Geometry check sheet. Reference: the model listing, model coordinates, mm. Face numbers are marked on the shaded views. A direction names the side the tool comes from. Give positions to 0.01 mm unless a question says otherwise; leave off trailing zeros. Loops run counter-clockwise (first coordinate to the right, second up) from the corner with the lowest first, then second, coordinate; pieces in that order, holes last. Notation, with made-up numbers: (62.25, -37.5) -> (82.25, -37.5) arc R20 cw to (82.25, -21.5) -> close; hole circle Ø10 at (60, 2). An arc over 180 degrees is marked (long way). One line per item, written item: value. Start each with the question number.
(1) Sectioned sample at C-C, the plane y = 42. Record the cut outline in (x, z).
(2) Sectioned sample at A-A, the plane x = 0. Record the cut outline in (y, z).
(3) Tool access check on the marked faces 1, 2 and 3. Record the directions out of +Z, -Z, +X, -X, +Y, -Y that give a thin tool (end or side, any length) a straight path to the whole face; none if there is none.
(4) Sectioned sample at B-B, the plane z = 0. Record the cut outline in (x, y).
(5) Scan lines: line 1 along Y through (x, z) = (6, -2.5); line 2 along X through (y, z) = (71.5, 0); line 3 along Y through (x, z) = (-3.5, -4). Record each from-to range of solid material in increasing order. Write a range as from..to.
(6) Sectioned sample at D-D, the plane z = 4. Record the cut outline in (x, y).
(7) Gauge pin test, flat ends, axial feed: pin 1 Ø5.5 at (x, z) = (-4, 3.5) entering from +Y; pin 2 Ø4 at (y, z) = (91.5, -0.5) entering from -X; pin 3 Ø6 at (x, y) = (2.5, 16) entering from -Z; pin 4 Ø1.5 at (x, y) = (-3.5, 87.5) entering from -Z. Record the tip position at first contact, or that the pin passes through.
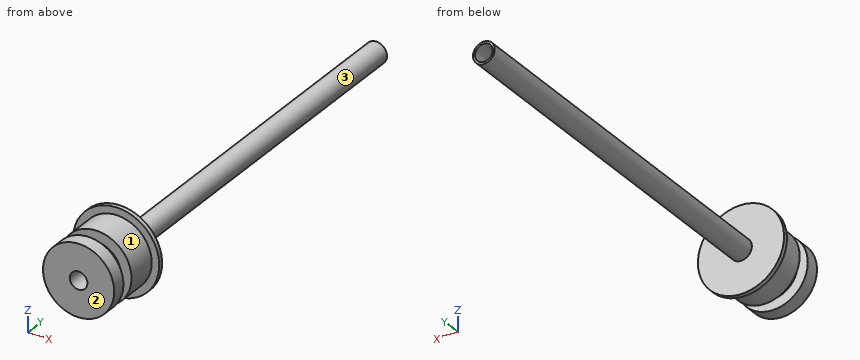
from build123d import *

# Parameters (mm, degrees)
SKETCH1_R           = 9.5
BOSS_EXTRUDE1_DEPTH = 14
SKETCH2_R           = 2.4
BOSS_EXTRUDE2_DEPTH = 89
SKETCH3_R           = 1.94
CUT_EXTRUDE1_DEPTH  = 104.872518021
SKETCH4_R           = 9.5
SKETCH4_R_2         = 7.85
CUT_EXTRUDE2_DEPTH  = 13
CUT_EXTRUDE3_START  = -3.2
SKETCH5_R           = 7.85
SKETCH5_R_2         = 5.55
CUT_EXTRUDE3_DEPTH  = 2.8


with BuildPart() as part:
    # Sketch1 → Boss-Extrude1 (new body)
    with BuildSketch(Plane(origin=(0, 0, 0), x_dir=(1, 0, 0), z_dir=(0, 1, 0))):
        with Locations(Location((0, 0, 0), (0, 0, 270))):
            Circle(SKETCH1_R)
    extrude(amount=BOSS_EXTRUDE1_DEPTH)

    # Sketch2 → Boss-Extrude2 (add)
    with BuildSketch(Plane(origin=(0, 14, 0), x_dir=(1, 0, 0), z_dir=(0, 1, 0))):
        with Locations(Location((0, 0, 0), (0, 0, 270))):
            Circle(SKETCH2_R)
    extrude(amount=BOSS_EXTRUDE2_DEPTH)

    # Sketch3 → Cut-Extrude1 (cut, through all)
    with BuildSketch(Plane(origin=(0, 103, 0), x_dir=(1, 0, 0), z_dir=(0, 1, 0))):
        with Locations(Location((0, 0, 0), (0, 0, 270))):
            Circle(SKETCH3_R)
    extrude(amount=-CUT_EXTRUDE1_DEPTH, mode=Mode.SUBTRACT)

    # Sketch4 → Cut-Extrude2 (cut)
    with BuildSketch(Plane.XZ):
        with Locations(Location((0, 0, 0), (0, 0, 270))):
            Circle(SKETCH4_R)
        with Locations(Location((0, 0, 0), (0, 0, 270))):
            Circle(SKETCH4_R_2, mode=Mode.SUBTRACT)
    extrude(amount=-CUT_EXTRUDE2_DEPTH, mode=Mode.SUBTRACT)

    # Sketch5 → Cut-Extrude3 (cut)
    with BuildSketch(Plane.XZ.offset(CUT_EXTRUDE3_START)):
        with Locations(Location((0, 0, 0), (0, 0, 270))):
            Circle(SKETCH5_R)
        with Locations(Location((0, 0, 0), (0, 0, 270))):
            Circle(SKETCH5_R_2, mode=Mode.SUBTRACT)
    extrude(amount=-CUT_EXTRUDE3_DEPTH, mode=Mode.SUBTRACT)


solid = part.part
Calculated:
1. outline: circle Ø4.8 at (0, 0); hole circle Ø3.88 at (0, 0)
2. outline: (0, -7.85) -> (3.2, -7.85) -> (3.2, -5.55) -> (6, -5.55) -> (6, -7.85) -> (13, -7.85) -> (13, -9.5) -> (14, -9.5) -> (14, -2.4) -> (103, -2.4) -> (103, -1.94) -> (0, -1.94) -> close; (0, 1.94) -> (103, 1.94) -> (103, 2.4) -> (14, 2.4) -> (14, 9.5) -> (13, 9.5) -> (13, 7.85) -> (6, 7.85) -> (6, 5.55) -> (3.2, 5.55) -> (3.2, 7.85) -> (0, 7.85) -> close
3. face 1: -Y
3. face 2: +Z, -Z, +X, -X, -Y
3. face 3: +Y
4. outline: (-9.5, 13) -> (-7.85, 13) -> (-7.85, 6) -> (-5.55, 6) -> (-5.55, 3.2) -> (-7.85, 3.2) -> (-7.85, 0) -> (-1.94, 0) -> (-1.94, 103) -> (-2.4, 103) -> (-2.4, 14) -> (-9.5, 14) -> close; (1.94, 0) -> (7.85, 0) -> (7.85, 3.2) -> (5.55, 3.2) -> (5.55, 6) -> (7.85, 6) -> (7.85, 13) -> (9.5, 13) -> (9.5, 14) -> (2.4, 14) -> (2.4, 103) -> (1.94, 103) -> close
5. line 1: y = 0..3.2, 6..14
5. line 2: x = -2.4..-1.94, 1.94..2.4
5. line 3: y = 0..14
6. outline: (-8.62, 13) -> (-6.75, 13) -> (-6.75, 6) -> (-3.85, 6) -> (-3.85, 3.2) -> (-6.75, 3.2) -> (-6.75, 0) -> (6.75, 0) -> (6.75, 3.2) -> (3.85, 3.2) -> (3.85, 6) -> (6.75, 6) -> (6.75, 13) -> (8.62, 13) -> (8.62, 14) -> (-8.62, 14) -> close
7. pin 1: stops at y = 14
7. pin 2: stops at x = -2.4
7. pin 3: stops at z = -9.5
7. pin 4: passes through
